```python
from build123d import *

# Parameters (mm, degrees)
F1_DEPTH    = 6.35
F2_T1_DEPTH = 97.79


# Not quite as in the source:
# - a fillet or chamfer that OpenCascade refuses, or shapes differently, is made with other operations: its cross-section is extruded or revolved along the edge and cut away or added


with BuildPart() as f1:
    # F0 (on Top) → F1 (new body)
    with BuildSketch(Plane.XY):
        with BuildLine():
            Line((-77.5854553002, 19.2668606828), (-77.5854553002, -15.0231393172))
            Line((-77.5854553002, -15.0231393172), (59.5745446998, -15.0231393172))
            Line((59.5745446998, -15.0231393172), (59.5745446998, 19.2668606828))
            Line((59.5745446998, 19.2668606828), (17.687636208, 19.2668606828))
            ThreePointArc((17.687636208, 19.2668606828), (1.177636208, 2.7568606828), (-15.332363792, 19.2668606828))
            Line((-15.332363792, 19.2668606828), (-60.4981811881, 19.2668606828))
            ThreePointArc((-60.4981811881, 19.2668606828), (-66.8481811881, 12.9168606828), (-73.1981811881, 19.2668606828))
            Line((-73.1981811881, 19.2668606828), (-77.5854553002, 19.2668606828))
        make_face()
        with BuildLine():
            Line((-77.5854553002, 53.5568606828), (-77.5854553002, 19.2668606828))
            Line((-77.5854553002, 19.2668606828), (-73.1981811881, 19.2668606828))
            ThreePointArc((-73.1981811881, 19.2668606828), (-66.8481811881, 25.6168606828), (-60.4981811881, 19.2668606828))
            Line((-60.4981811881, 19.2668606828), (-15.332363792, 19.2668606828))
            ThreePointArc((-15.332363792, 19.2668606828), (1.177636208, 35.7768606828), (17.687636208, 19.2668606828))
            Line((17.687636208, 19.2668606828), (59.5745446998, 19.2668606828))
            Line((59.5745446998, 19.2668606828), (59.5745446998, 53.5568606828))
            Line((59.5745446998, 53.5568606828), (-77.5854553002, 53.5568606828))
        make_face()
    extrude(amount=F1_DEPTH)

    # F2: fillet of radius 5.842 on 1 edges, made by hand

    # F2_s2 → F2_t1 (cut)
    with BuildSketch(Plane.XZ.offset(-68.1618606828)):
        with BuildLine():
            ThreePointArc((-77.5854553002, 0.508), (-75.8743731159, 4.6389178157), (-71.7434553002, 6.35))
            Line((-71.7434553002, 6.35), (-77.5854553002, 6.35))
            Line((-77.5854553002, 6.35), (-77.5854553002, 0.508))
        make_face()
    extrude(amount=F2_T1_DEPTH, mode=Mode.SUBTRACT)


solid = f1.part
```
Verification items for the finished model (mm, model axes). Give positions to 0.01 mm unless a question says otherwise; leave off trailing zeros. Loops run counter-clockwise (first coordinate to the right, second up) from the corner with the lowest first, then second, coordinate; pieces in that order, holes last.
1. Section check A-A, the plane y = 10. Enter the section's corners in (x, z).
2. Thickness scan on line 1 (X direction, y = 14, z = 2) (3 decimals); line 2 (X direction, y = 41, z = 0.75); line 3 (X direction, y = 22.5, z = 2.25). Record the ranges inside material, lowest first.
3. Mould release check, pull along X, two halves, no side actions. Record for faces 1 (the flat face through (-25, 20, 0)), 2 (the cylindrical face through (-69.778, 13.633, 3.131)), 3 (the cylindrical face through (-75.92, 19.75, 4.59)), 4 (the flat face through (59.575, 19, 3)): released by +X, released by -X, zero draft, split by the parting line, or undercut.
4. Section check B-B, the plane x = 0. Enter the section's corners in (y, z), then the cut area to 3 significant figures.
5. Section check C-C, the plane z = 3. Enter the section's corners in (x, y).
6. Section check D-D, the plane y = 28. Enter the section's corners in (x, z).
Geometry says:
1. outline: (-77.59, 0) - (-12.49, 0) - (-12.49, 6.35) - (-71.74, 6.35) arc R5.84 ccw to (-77.59, 0.51) - close; (14.84, 0) - (59.57, 0) - (59.57, 6.35) - (14.84, 6.35) - close
2. line 1: x = -77.392 to -70.395, -63.301 to -14.47, 16.825 to 59.575
2. line 2: x = -77.58 to 59.57
2. line 3: x = -77.32 to -72.31, -61.38 to -15.01, 17.37 to 59.57
3. face 1: zero draft
3. face 2: undercut
3. face 3: released by -X
3. face 4: released by +X
4. outline: (-15.02, 0) - (2.8, 0) - (2.8, 6.35) - (-15.02, 6.35) - close; (35.73, 0) - (53.56, 0) - (53.56, 6.35) - (35.73, 6.35) - close
4. area: 226 mm2
5. outline: (-77.03, -15.02) - (59.57, -15.02) - (59.57, 53.56) - (-77.03, 53.56) - close; hole circle Ø12.7 at (-66.85, 19.27); hole circle Ø33.02 at (1.18, 19.27)
6. outline: (-77.59, 0) - (-12.83, 0) - (-12.83, 6.35) - (-71.74, 6.35) arc R5.84 ccw to (-77.59, 0.51) - close; (15.19, 0) - (59.57, 0) - (59.57, 6.35) - (15.19, 6.35) - close
